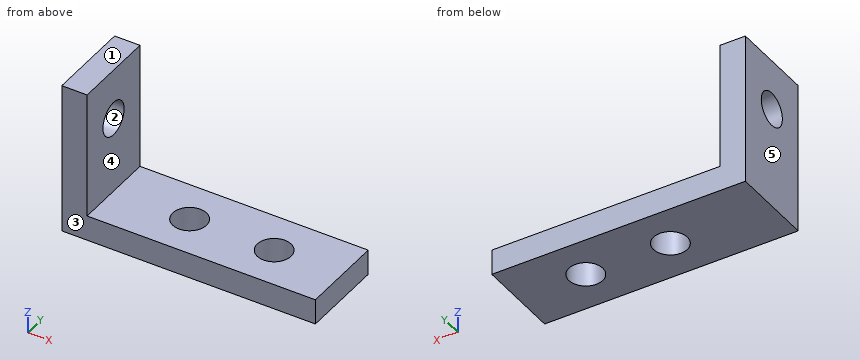
from build123d import *

# Parameters (mm, degrees)
SKETCH2_W           = 30
SKETCH2_H           = 10
SKETCH2_R           = 2
BOSS_EXTRUDE1_DEPTH = 3
SKETCH3_W           = 3
SKETCH3_H           = 10
BOSS_EXTRUDE2_DEPTH = 15
SKETCH4_R           = 2
CUT_EXTRUDE1_DEPTH  = 27


with BuildPart() as part:
    # Sketch2 → Boss-Extrude1 (new body)
    with BuildSketch(Plane.XY):
        with Locations((15, 5)):
            Rectangle(SKETCH2_W, SKETCH2_H)
        with Locations((12, 5)):
            Circle(SKETCH2_R, mode=Mode.SUBTRACT)
        with Locations((22, 5)):
            Circle(SKETCH2_R, mode=Mode.SUBTRACT)
    extrude(amount=BOSS_EXTRUDE1_DEPTH)

    # Sketch3 → Boss-Extrude2 (add)
    with BuildSketch(Plane.XY.offset(3)):
        with Locations((1.5, 5)):
            Rectangle(SKETCH3_W, SKETCH3_H)
    extrude(amount=BOSS_EXTRUDE2_DEPTH)

    # Sketch4 → Cut-Extrude1 (cut)
    with BuildSketch(Plane(origin=(3, 0, 0), x_dir=(0, 0, -1), z_dir=(1, 0, 0))):
        with Locations((-22, 5)):
            Circle(SKETCH4_R)
        with Locations(Location((-12, 5, 0), (0, 0, 90))):
            Circle(SKETCH4_R)
    extrude(amount=-CUT_EXTRUDE1_DEPTH, mode=Mode.SUBTRACT)


solid = part.part
Source: CAD feature listing. Evaluate the final solid. Frame: model axes, mm. Face numbers are marked on the shaded views. A direction names the side the tool comes from. Coordinates: 2 decimals unless noted, no trailing zeros. Order: outer loops, then holes, each group sorted by start corner. A loop starts at its lowest first (then second) coordinate and runs counter-clockwise, first axis right, second up.
Item 1: Set-up query: the marked faces 4 and 5. Return all of +Z, -Z, +X, -X, +Y, -Y with unobstructed straight access to the full face (end or side cutting, diameter ignored); none if empty.
Output values:
face 4: +Z, +X, +Y, -Y
face 5: +Z, -Z, -X, +Y, -Y
Item 2: Material intervals for line 1 (Y direction, x = 12, z = 1.55); line 2 (Z direction, x = 9, y = 7.75), sorted ascending.
Output values:
line 1: y = 0 to 3, 7 to 10
line 2: z = 0 to 3
Item 3: Pull-direction query (Y, two-part tool) for the marked faces 1, 2 and 3; classes: pulls with the +Y half, pulls with the -Y half, needs draft (parallel to the pull), parting line crosses it, or undercut.
Output values:
face 1: needs draft
face 2: undercut
face 3: pulls with the -Y half
Item 4: Cut plane D-D (z = 2.5). Return loops of the section in (x, y).
Output values:
outline: (0, 0) - (30, 0) - (30, 10) - (0, 10) - close; hole circle Ø4 at (12, 5); hole circle Ø4 at (22, 5)
Item 5: Cut plane C-C (z = 12). Return loops of the section in (x, y).
Output values:
outline: (0, 0) - (3, 0) - (3, 3) - (0, 3) - close; (0, 7) - (3, 7) - (3, 10) - (0, 10) - close
Item 6: First-contact query: P1, Ø10, axis at x = 13, z = 10, coming from the +Y side; P2, Ø5, axis at x = 18, y = 4.5, coming from the +Z side; P3, Ø5, axis at y = 3, z = 7.5, coming from the +X side. Flat tips, straight axial feed; report the tip coordinate or a pass-through.
Output values:
P1: passes through
P2: stops at z = 3
P3: stops at x = 3
Item 7: Cut plane A-A (x = 12). Return loops of the section in (y, z).
Output values:
outline: (0, 0) - (3, 0) - (3, 3) - (0, 3) - close; (7, 0) - (10, 0) - (10, 3) - (7, 3) - close
Item 8: Cut plane B-B (y = 5). Return loops of the section in (x, z).
Output values:
outline: (0, 0) - (10, 0) - (10, 3) - (3, 3) - (3, 10) - (0, 10) - close; (0, 14) - (3, 14) - (3, 18) - (0, 18) - close; (14, 0) - (20, 0) - (20, 3) - (14, 3) - close; (24, 0) - (30, 0) - (30, 3) - (24, 3) - close
